Could you check a few things on this drawing? It's one solid part, dimensions in mm from its lowest x, y, z. A direction names the side the tool comes from. Give positions to 0.01 mm unless a question says otherwise; leave off trailing zeros. Loops run counter-clockwise (first coordinate to the right, second up) from the corner with the lowest first, then second, coordinate; pieces in that order, holes last. Notation, with made-up numbers: (64.5, 49) - (96.5, 49) arc R18 cw to (96.5, 53) - close; hole circle Ø7 at (-5.5, 84.5). An arc over 180 degrees is marked (long way). Return JSON: item names as keys, results as strings. Group by question number.
(1) I need wall thicknesses on probe 1 along Z at (x, y) = (6.75, 11); probe 2 along Y at (x, z) = (21, 1.2). Which ranges of each line are inside material? Lowest first, please. Write a range as [from, to].
(2) If we mould it in two halves opening along Z, with no side actions, what happens to the marked faces 3, 4 and 5? For each: released by +Z, released by -Z, zero draft, split by the parting line, or undercut.
(3) If we section it at C-C (x = 21): Please give me the cut outline in (y, z), then the cut area to 3 significant figures.
(4) If we section it at A-A (y = 10): Please give me the cut outline in (x, z).
(5) If we section it at D-D (y = 2): Please give me the cut outline in (x, z), then the cut area to 3 significant figures.
(6) For P1, Ø3, axis at y = 2.5, z = 18.5, coming from the +X side; P2, Ø3, axis at x = 7.5, y = 13, coming from the +Z side, each with a flat end and sliding along its axis, tell me the tip position at first contact or that it passes through.
(7) If we section it at B-B (z = 10): Please give me the cut outline in (x, y), then the cut area to 3 significant figures.
(8) On a 3-axis mill with a long thin cutter (end or side, diameter ignored), from which of +Z, -Z, +X, -X, +Y, -Y can I reach the whole of each face in a straight line? I mean the marked faces 1 and 2. Say none if no direction works.
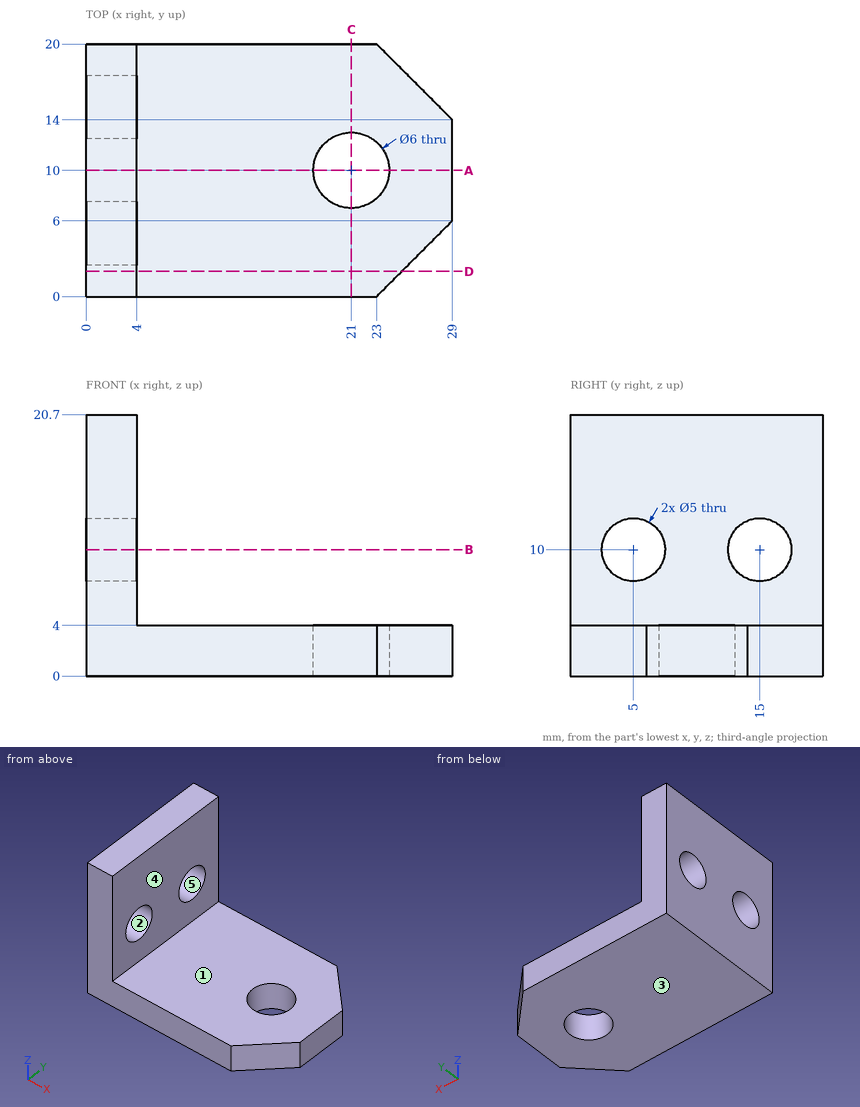
Values:
{
 "1": {"probe 1": "[0, 4]", "probe 2": "[0, 7], [13, 20]"},
 "2": {"face 3": "released by -Z", "face 4": "zero draft", "face 5": "undercut"},
 "3": {"outline": "(0, 0) - (7, 0) - (7, 4) - (0, 4) - close; (13, 0) - (20, 0) - (20, 4) - (13, 4) - close", "area": "56.0 mm2"},
 "4": {"outline": "(0, 0) - (18, 0) - (18, 4) - (4, 4) - (4, 20.7) - (0, 20.7) - close; (24, 0) - (29, 0) - (29, 4) - (24, 4) - close"},
 "5": {"outline": "(0, 0) - (25, 0) - (25, 4) - (4, 4) - (4, 20.7) - (0, 20.7) - close", "area": "167 mm2"},
 "6": {"P1": "x = 4", "P2": "z = 4"},
 "7": {"outline": "(0, 0) - (4, 0) - (4, 2.5) - (0, 2.5) - close; (0, 7.5) - (4, 7.5) - (4, 12.5) - (0, 12.5) - close; (0, 17.5) - (4, 17.5) - (4, 20) - (0, 20) - close", "area": "40.0 mm2"},
 "8": {"face 1": "+Z, +X, +Y, -Y", "face 2": "+X, -X"}
}
